Drawing for the job (mm, zero at the part's lowest x, y, z). Give positions to 0.01 mm unless a question says otherwise; leave off trailing zeros. Loops run counter-clockwise (first coordinate to the right, second up) from the corner with the lowest first, then second, coordinate; pieces in that order, holes last. Notation, with made-up numbers: (14.25, 48) -> (72.25, 48) arc R11 ccw to (72.25, 67) -> close; hole circle Ø10 at (-21, -25.75). An arc over 180 degrees is marked (long way). Write item = value, one per line.
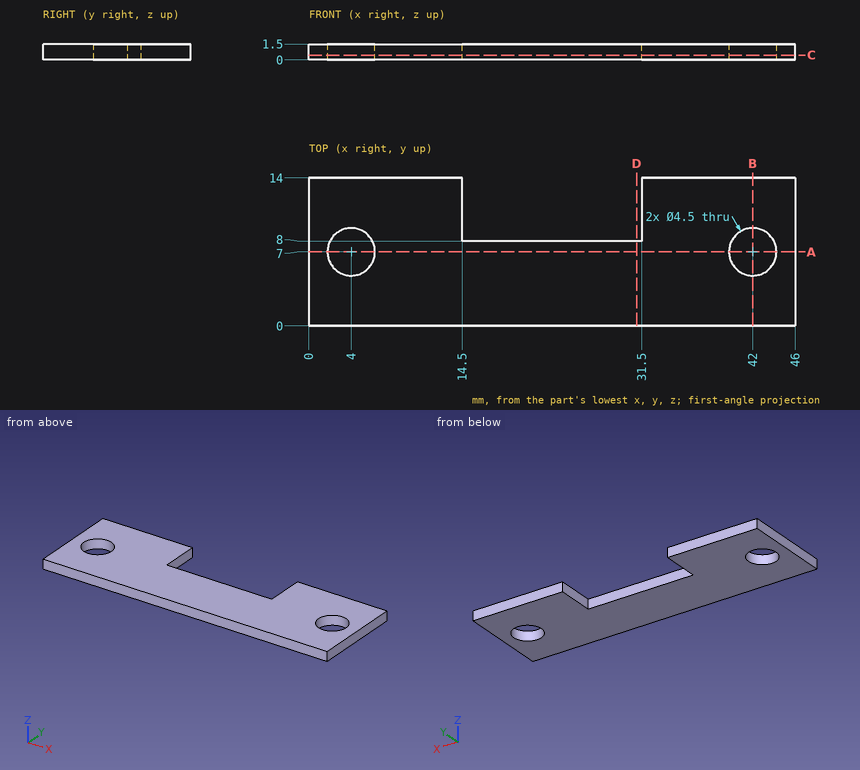
1) Slice it at A-A, the plane y = 7. List the corners of the cut face in (x, z), and give its area (3 significant figures).
Resolved:
outline = (0, 0) -> (1.75, 0) -> (1.75, 1.5) -> (0, 1.5) -> close; (6.25, 0) -> (39.75, 0) -> (39.75, 1.5) -> (6.25, 1.5) -> close; (44.25, 0) -> (46, 0) -> (46, 1.5) -> (44.25, 1.5) -> close
area = 55.5 mm²
2) Drop a flat-ended pin along its axis: P1, Ø7, axis at x = 4, y = 7, coming from the -Z side. Give the stop position or say it passes through.
Resolved:
P1 = 0
3) Slice it at C-C, the plane z = 0.45. List the corners of the cut face in (x, y).
Resolved:
outline = (0, 0) -> (46, 0) -> (46, 14) -> (31.5, 14) -> (31.5, 8) -> (14.5, 8) -> (14.5, 14) -> (0, 14) -> close; hole circle Ø4.5 at (4, 7); hole circle Ø4.5 at (42, 7)
4) Slice it at D-D, the plane x = 31. List the corners of the cut face in (y, z).
Resolved:
outline = (0, 0) -> (8, 0) -> (8, 1.5) -> (0, 1.5) -> close
5) Slice it at B-B, the plane x = 42. List the corners of the cut face in (y, z), and give its area (4 significant figures).
Resolved:
outline = (0, 0) -> (4.75, 0) -> (4.75, 1.5) -> (0, 1.5) -> close; (9.25, 0) -> (14, 0) -> (14, 1.5) -> (9.25, 1.5) -> close
area = 14.25 mm²
6) Drill centre lines: line 1 along X through (y, z) = (10.5, 0.7); line 2 along Y through (x, z) = (42, 0.7); line 3 along X through (y, z) = (7.75, 0.65). Where is each one in solid material? Low to high. Write a range as [from, to].
Resolved:
line_1 = [0, 14.5], [31.5, 46]
line_2 = [0, 4.75], [9.25, 14]
line_3 = [0, 1.88], [6.12, 39.88], [44.12, 46]
